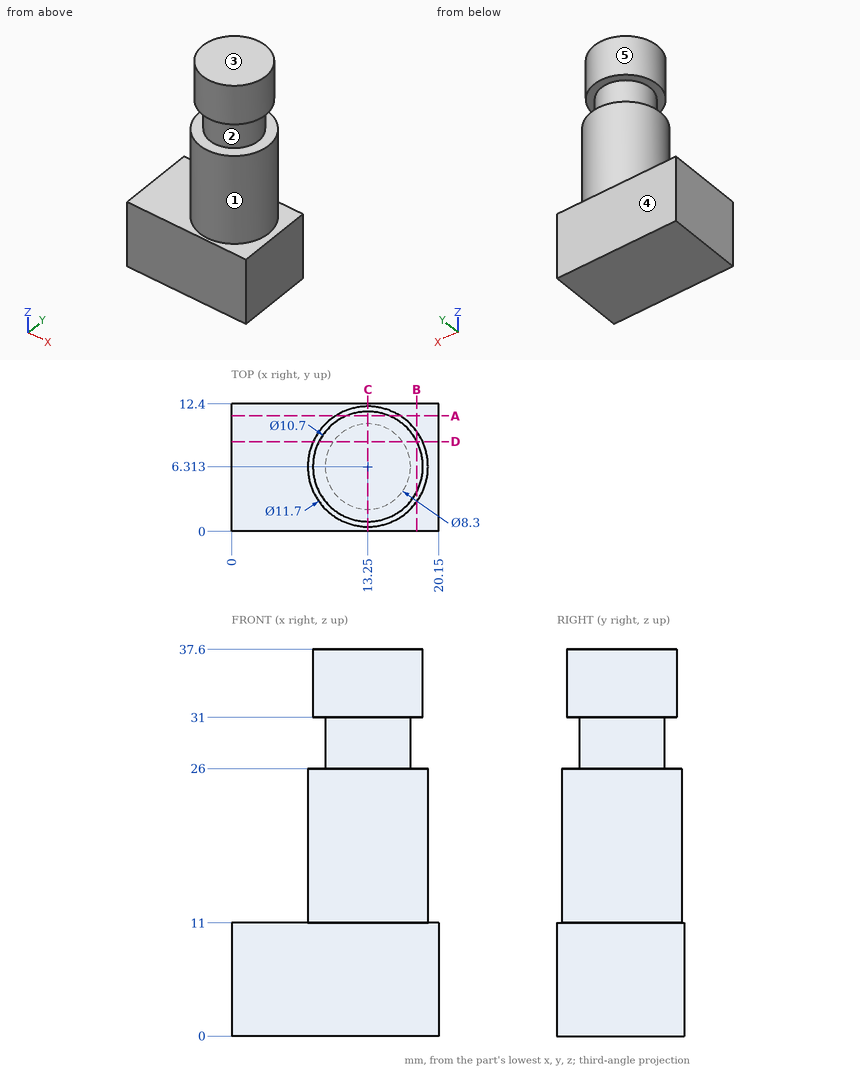
Input: dimensioned drawing with shaded views. Units: mm. Origin: part minimum x, y, z. A direction names the side the tool comes from. Round coordinates to 2 decimals unless told otherwise and drop trailing zeros. Loops run counter-clockwise (first coordinate to the right, second up) from the corner with the lowest first, then second, coordinate; pieces in that order, holes last. Notation, with made-up numbers: (28.5, 44) -> (85.5, 44) arc R37 cw to (85.5, 80) -> close; hole circle Ø3 at (74.25, -8.75). An arc over 180 degrees is marked (long way). Answer as a JSON object with one key per item and string values. Group by question number.
1) Reachability of the marked faces 4 and 5 from +Z, -Z, +X, -X, +Y, -Y: full face, straight path, thin tool, end or side. Return the list, or none.
2) Section query C-C on x = 13.25. Output: boundary loops of the cut face in (y, z).
3) Section query A-A on y = 11.25. Output: boundary loops of the cut face in (x, z), plus the area to 3 significant figures.
4) Pin query (flat end, axial travel): pin 1 (3 mm diameter, centred on y = 6.5, z = 27, fed in from -X); pin 2 (8 mm diameter, centred on x = 3.5, z = 11, fed in from -Y); pin 3 (2 mm diameter, centred on x = 12.5, z = 18, fed in from -Y); pin 4 (5 mm diameter, centred on y = 9, z = 30, fed in from -X). Return the tip coordinate at first contact, or that it passes through.
5) Section query D-D on y = 8.75. Output: boundary loops of the cut face in (x, z), plus the area to 3 significant figures.
6) Draft query along Z for the marked faces 1, 2 and 3. Return one class per face: +Z half, -Z half, draft (parallel to the pull), parting line (faces both ways), or undercut.
7) Section query B-B on x = 18. Output: boundary loops of the cut face in (y, z) (1 decimal).
8) Ray query, L1, parallel to Z at x = 16.25, y = 2.75; L2, parallel to Z at x = 18.5, y = 8; L3, parallel to Z at x = 6.5, y = 3. Return the intervals inside material, ascending.
Reply:
{
 "1": {"face 4": "+Z, -Z, +X, -X, +Y", "face 5": "+Z"},
 "2": {"outline": "(0, 0) -> (12.4, 0) -> (12.4, 11) -> (12.16, 11) -> (12.16, 26) -> (10.46, 26) -> (10.46, 31) -> (11.66, 31) -> (11.66, 37.6) -> (0.96, 37.6) -> (0.96, 31) -> (2.16, 31) -> (2.16, 26) -> (0.46, 26) -> (0.46, 11) -> (0, 11) -> close"},
 "3": {"outline": "(0, 0) -> (20.15, 0) -> (20.15, 11) -> (16.39, 11) -> (16.39, 26) -> (10.11, 26) -> (10.11, 11) -> (0, 11) -> close; (11.19, 31) -> (15.31, 31) -> (15.31, 37.6) -> (11.19, 37.6) -> close", "area": "343 mm2"},
 "4": {"pin 1": "stops at x = 7.4", "pin 2": "stops at y = 0", "pin 3": "stops at y = 0.46", "pin 4": "stops at x = 7.91"},
 "5": {"outline": "(0, 0) -> (20.15, 0) -> (20.15, 11) -> (18.57, 11) -> (18.57, 26) -> (16.61, 26) -> (16.61, 31) -> (18.01, 31) -> (18.01, 37.6) -> (8.49, 37.6) -> (8.49, 31) -> (9.89, 31) -> (9.89, 26) -> (7.93, 26) -> (7.93, 11) -> (0, 11) -> close", "area": "478 mm2"},
 "6": {"face 1": "draft", "face 2": "undercut", "face 3": "+Z half"},
 "7": {"outline": "(0, 0) -> (12.4, 0) -> (12.4, 11) -> (9.7, 11) -> (9.7, 26) -> (2.9, 26) -> (2.9, 11) -> (0, 11) -> close; (3.9, 31) -> (8.8, 31) -> (8.8, 37.6) -> (3.9, 37.6) -> close"},
 "8": {"L1": "z = 0 to 26, 31 to 37.6", "L2": "z = 0 to 26", "L3": "z = 0 to 11"}
}
